```python
from build123d import *

# Parameters (mm, degrees)
SKETCH1_W           = 457.2
SKETCH1_H           = 304.8
CHAMBER_BASE_DEPTH  = 457.2
SKETCH2_W           = 457.2
SKETCH2_H           = 304.8
BACK_WALL_DEPTH     = 6.35
SKETCH3_W           = 463.55
SKETCH3_H           = 457.2
SIDE_WALL_2_DEPTH   = 6.35
SKETCH5_W           = 463.55
SKETCH5_H           = 457.2
SIDE_WALL_3_DEPTH   = 6.35
SKETCH8_W           = 463.55
SKETCH8_H           = 317.5
TOP_DEPTH           = 6.35
SKETCH9_R           = 38.1
BOSS_EXTRUDE1_DEPTH = 50.8
SKETCH10_R          = 50.8
BOSS_EXTRUDE2_DEPTH = 25.4
SKETCH11_R          = 1.5875
BOSS_EXTRUDE3_DEPTH = 50.8


with BuildPart() as part:
    # Sketch1 → Chamber Base (new body)
    with BuildSketch(Plane.XY):
        with Locations((228.6, 152.4)):
            Rectangle(SKETCH1_W, SKETCH1_H)
    extrude(amount=CHAMBER_BASE_DEPTH)

    # Sketch2 → Back wall (add)
    with BuildSketch(Plane(origin=(457.2, 0, 0), x_dir=(0, 0, -1), z_dir=(1, 0, 0))):
        with Locations((-228.6, 152.4)):
            Rectangle(SKETCH2_W, SKETCH2_H)
    extrude(amount=BACK_WALL_DEPTH)

    # Sketch3 → Side wall 2 (add)
    with BuildSketch(Plane(origin=(0, 304.8, 0), x_dir=(1, 0, 0), z_dir=(0, 1, 0))):
        with Locations((231.775, -228.6)):
            Rectangle(SKETCH3_W, SKETCH3_H)
    extrude(amount=SIDE_WALL_2_DEPTH)

    # Sketch5 → Side wall 3 (add)
    with BuildSketch(Plane.XZ):
        with Locations((231.775, 228.6)):
            Rectangle(SKETCH5_W, SKETCH5_H)
    extrude(amount=SIDE_WALL_3_DEPTH)

    # Sketch8 → Top (add)
    with BuildSketch(Plane.XY.offset(457.2)):
        with Locations((231.775, 152.4)):
            Rectangle(SKETCH8_W, SKETCH8_H)
    extrude(amount=TOP_DEPTH)

    # Sketch9 → Boss-Extrude1 (add)
    with BuildSketch(Plane.XY.offset(463.55)):
        with Locations((231.775, 152.4)):
            Circle(SKETCH9_R)
    extrude(amount=BOSS_EXTRUDE1_DEPTH)

    # Sketch10 → Boss-Extrude2 (add)
    with BuildSketch(Plane(origin=(0, 0, 0), x_dir=(-1, 0, 0), z_dir=(0, 0, -1))):
        with Locations((-231.775, 152.4)):
            Circle(SKETCH10_R)
    extrude(amount=BOSS_EXTRUDE2_DEPTH)

    # Sketch11 → Boss-Extrude3 (add)
    with BuildSketch(Plane.XY.offset(514.35)):
        with Locations((231.775, 152.4)):
            Circle(SKETCH11_R)
    extrude(amount=BOSS_EXTRUDE3_DEPTH)

    # Sketch15 → Revolve1 (revolve)
    with BuildSketch(Plane.ZY.offset(-231.775)):
        Polygon((514.35, 190.5), (514.35, 152.4), (565.15, 152.4), align=None)
    revolve(axis=Axis((231.775, 152.4, 514.35), (0, 0, 1)))


solid = part.part
```
Geometry check sheet. Reference: the model listing, model coordinates, mm. A direction names the side the tool comes from. Give positions to 0.01 mm unless a question says otherwise; leave off trailing zeros. Loops run counter-clockwise (first coordinate to the right, second up) from the corner with the lowest first, then second, coordinate; pieces in that order, holes last. Notation, with made-up numbers: M -14.5,10.5 L 33.5,10.5 A21 cw 33.5,34.5 Z; hole C 30,45 d6. An arc over 180 degrees is marked long. Answer as CSV lines item,"result".
Item 1: Material ranges on line 1 (Z direction, x = 61.5, y = 199), recorded low to high.
Values:
line 1,"z = 0 to 463.55"
Item 2: Cross-section at B-B on y = 235.5. Record the cut outline in (x, z).
Values:
outline,"M 0,0 L 463.55,0 L 463.55,463.55 L 0,463.55 Z"
Item 3: Access from +Z, -Z, +X, -X, +Y, -Y to the whole of each face (thin tool, end or side, straight path). Record for faces 1 (the cylindrical face through (203.694, 178.15, 488.594)), 2 (the cylindrical face through (282.526, 154.634, -12.522)), 3 (the flat face through (229, 311.15, 229)).
Values:
face 1,"+Z"
face 2,"-Z"
face 3,"+Z, -Z, +X, -X, +Y"
Item 4: Cross-section at A-A on z = 478. Record the cut outline in (x, y) (3 decimals), and give its area (3 significant figures).
Values:
outline,"C 231.775,152.4 d76.2"
area,"4,560 mm²"
Item 5: Depth check by flat-ended pin: P1, Ø6, axis at x = 262.5, y = 176.5, coming from the +Z side; P2, Ø10, axis at y = 199, z = 475.5, coming from the +X side; P3, Ø12, axis at x = 84, y = 120.5, coming from the -Z side. Enter the tip coordinate at first touch or a pass-through.
Values:
P1,"stops at z = 517.08"
P2,"passes through"
P3,"stops at z = 0"
Item 6: Cross-section at C-C on x = 324. Record the cut outline in (y, z), and give its area (3 significant figures).
Values:
outline,"M -6.35,0 L 311.15,0 L 311.15,463.55 L -6.35,463.55 Z"
area,"147,000 mm²"
